from build123d import *

# Parameters (mm, degrees)
BOSS_EXTRUDE1_DEPTH             = 2.54
BOSS_EXTRUDE1_DEPTH_BACK        = 2.54
BOSS_EXTRUDE2_REACH             = 44.034
SKETCH2_R                       = 6.35
BOSS_EXTRUDE2_DIRECTION_2_DEPTH = 1.016
BOSS_EXTRUDE3_DEPTH             = 1.016
BOSS_EXTRUDE3_DEPTH_BACK        = 4.7625
SKETCH3_R                       = 6.35
CUT_EXTRUDE1_DEPTH              = 46.159171383
CUT_EXTRUDE1_DEPTH_BACK         = 46.159171383
BOSS_EXTRUDE4_DEPTH             = 6.35
BOSS_EXTRUDE4_DEPTH_BACK        = 6.35
CUT_EXTRUDE2_DEPTH              = 46.159171383
CUT_EXTRUDE2_DEPTH_BACK         = 46.159171383
SKETCH7_R                       = 0.79375
FILLET1_R                       = 12.7
FILLET2_R                       = 15.875
FILLET3_R                       = 25.4
CUT_EXTRUDE3_DEPTH              = 39.905968649
CUT_EXTRUDE3_DEPTH_BACK         = 39.905968649
SKETCH8_R                       = 2.413


with BuildPart() as part:
    # Sketch1 → Boss-Extrude1 (new, two sides: drawn at the far end of the back side and taken through both)
    with BuildSketch(Plane(origin=(0, 0, 0), x_dir=(1, 0, 0), z_dir=(0, 1, 0)).offset(-BOSS_EXTRUDE1_DEPTH_BACK)):
        with BuildLine():
            Line((-13.716, 6.35), (-8.9535, 6.35))
            Line((-8.9535, 6.35), (-8.9535, -9.525))
            Line((-8.9535, -9.525), (-2.772279089, -20.597609011))
            ThreePointArc((-2.772279089, -20.597609011), (0, -22.225), (2.772279089, -20.597609011))
            Line((2.772279089, -20.597609011), (8.9535, -9.525))
            Line((8.9535, -9.525), (8.9535, 6.35))
            Line((8.9535, 6.35), (13.716, 6.35))
            Line((13.716, 6.35), (13.716, -15.944447946))
            Line((13.716, -15.944447946), (4.32475538, -32.767270057))
            ThreePointArc((4.32475538, -32.767270057), (0, -35.306), (-4.32475538, -32.767270057))
            Line((-4.32475538, -32.767270057), (-13.716, -15.944447946))
            Line((-13.716, -15.944447946), (-13.716, 6.35))
        make_face()
    extrude(amount=BOSS_EXTRUDE1_DEPTH + BOSS_EXTRUDE1_DEPTH_BACK)

    # Boss-Extrude2: up to this face of the body (flat: up to its plane)
    boss_extrude2_end = Plane(part.part.faces().sort_by_distance((-13.716, 0, 4.797223973))[0])
    # Sketch2 → Boss-Extrude2 (add, up to the picked face)
    with BuildSketch(Plane(origin=(-8.9535, 0, 0), x_dir=(0, 0, -1), z_dir=(1, 0, 0)), mode=Mode.PRIVATE) as boss_extrude2_sk1:
        Circle(SKETCH2_R)
    boss_extrude2_tool1 = split(extrude(boss_extrude2_sk1.sketch, amount=-BOSS_EXTRUDE2_REACH, mode=Mode.PRIVATE), bisect_by=boss_extrude2_end, keep=Keep.BOTH, mode=Mode.PRIVATE)
    add(boss_extrude2_tool1.solids().sort_by(Axis((-8.9535, 0, 0), (-1, 0, 0)))[0])

    # Sketch2 → Boss-Extrude2 direction 2 (add)
    with BuildSketch(Plane(origin=(-8.9535, 0, 0), x_dir=(0, 0, -1), z_dir=(1, 0, 0))):
        Circle(SKETCH2_R)
    extrude(amount=BOSS_EXTRUDE2_DIRECTION_2_DEPTH)

    # Sketch3 → Boss-Extrude3 (add, two sides: drawn at the far end of the back side and taken through both)
    with BuildSketch(Plane.ZY.offset(-8.9535).offset(-BOSS_EXTRUDE3_DEPTH_BACK)):
        with Locations(Location((0, 0, 0), (0, 0, 180))):
            Circle(SKETCH3_R)
    extrude(amount=BOSS_EXTRUDE3_DEPTH + BOSS_EXTRUDE3_DEPTH_BACK)

    # Sketch4 → Cut-Extrude1 (cut, two sides: drawn at the far end of the back side and taken through both)
    with BuildSketch(Plane(origin=(13.716, 0, 0), x_dir=(0, 0, -1), z_dir=(1, 0, 0)).offset(-CUT_EXTRUDE1_DEPTH_BACK)):
        with BuildLine():
            Line((3.81, 5.08), (13.97, 5.08))
            Line((13.97, 5.08), (13.97, -5.08))
            Line((13.97, -5.08), (3.81, -5.08))
            ThreePointArc((3.81, -5.08), (6.35, 0), (3.81, 5.08))
        make_face()
    extrude(amount=CUT_EXTRUDE1_DEPTH + CUT_EXTRUDE1_DEPTH_BACK, mode=Mode.SUBTRACT)

    # Sketch6 → Boss-Extrude4 (add, two sides: drawn at the far end of the back side and taken through both)
    with BuildSketch(Plane(origin=(0, 0, 0), x_dir=(1, 0, 0), z_dir=(0, 1, 0)).offset(-BOSS_EXTRUDE4_DEPTH_BACK)):
        with BuildLine():
            Line((-8.9535, -9.525), (-2.772279089, -20.597609011))
            ThreePointArc((-2.772279089, -20.597609011), (0, -22.225), (2.772279089, -20.597609011))
            Line((2.772279089, -20.597609011), (8.9535, -9.525))
            Line((8.9535, -9.525), (8.9535, 0))
            Line((8.9535, 0), (12.1285, 0))
            Line((12.1285, 0), (12.1285, -10.351202795))
            Line((12.1285, -10.351202795), (5.544558179, -22.145218022))
            ThreePointArc((5.544558179, -22.145218022), (0, -25.4), (-5.544558179, -22.145218022))
            Line((-5.544558179, -22.145218022), (-12.1285, -10.351202795))
            Line((-12.1285, -10.351202795), (-12.1285, 0))
            Line((-12.1285, 0), (-8.9535, 0))
            Line((-8.9535, 0), (-8.9535, -9.525))
        make_face()
    extrude(amount=BOSS_EXTRUDE4_DEPTH + BOSS_EXTRUDE4_DEPTH_BACK)

    # Sketch7 → Cut-Extrude2 (cut, two sides: drawn at the far end of the back side and taken through both)
    with BuildSketch(Plane(origin=(13.716, 0, 0), x_dir=(0, 0, -1), z_dir=(1, 0, 0)).offset(-CUT_EXTRUDE2_DEPTH_BACK)):
        Circle(SKETCH7_R)
    extrude(amount=CUT_EXTRUDE2_DEPTH + CUT_EXTRUDE2_DEPTH_BACK, mode=Mode.SUBTRACT)

    # Fillet1
    fillet1_edges = [part.edges().sort_by_distance(p)[0] for p in [
        (-8.9535, 0, 9.525),
        (8.9535, 0, 9.525),
    ]]
    fillet(fillet1_edges, radius=FILLET1_R)

    # Fillet2
    fillet2_edges = [part.edges().sort_by_distance(p)[0] for p in [
        (-12.1285, -4.445, 10.351202795),
        (12.1285, -4.445, 10.351202795),
        (-12.1285, 4.445, 10.351202795),
        (12.1285, 4.445, 10.351202795),
    ]]
    fillet(fillet2_edges, radius=FILLET2_R)

    # Fillet3
    fillet3_edges = [part.edges().sort_by_distance(p)[0] for p in [
        (13.716, 0, 15.944447946),
        (-13.716, 0, 15.944447946),
    ]]
    fillet(fillet3_edges, radius=FILLET3_R)

    # Sketch8 → Cut-Extrude3 (cut, two sides: drawn at the far end of the back side and taken through both)
    with BuildSketch(Plane(origin=(0, 2.54, 0), x_dir=(1, 0, 0), z_dir=(0, 1, 0)).offset(-CUT_EXTRUDE3_DEPTH_BACK)):
        with Locations(Location((0, -30.353, 0), (0, 0, 270))):
            Circle(SKETCH8_R)
    extrude(amount=CUT_EXTRUDE3_DEPTH + CUT_EXTRUDE3_DEPTH_BACK, mode=Mode.SUBTRACT)


solid = part.part
Input: part model. Units: mm. Frame: model coordinates. A direction names the side the tool comes from. Round coordinates to 2 decimals unless told otherwise and drop trailing zeros. Write each loop counter-clockwise with the first axis right and the second up, starting at its lowest first coordinate (ties: lowest second). Pieces come first, ordered by that corner, then holes.
1) Cut plane C-C (x = 6.5). Return the cut outline in (y, z), then the cut area to 3 significant figures.
2) Draft query along Y for faces 1 (the flat face through (-8.954, 5, 5)), 2 (the cylindrical face through (-10.867, -0.775, 0.172)), 3 (the flat face through (0, -2.54, 26)). Return one class per face: pulls with the +Y half, pulls with the -Y half, needs draft (parallel to the pull), parting line crosses it, or undercut.
3) Cut plane B-B (z = 14.5). Return the cut outline in (x, y), then the cut area to 3 significant figures.
4) Reachability of faces 4 (the cylindrical face through (-11.63, -4.42, 10.16)), 5 (the flat face through (-5.09, -0.089, 16.445)), 6 (the flat face through (-8.954, -5, 5)), 7 (the flat face through (8.954, 5, 5)) from +Z, -Z, +X, -X, +Y, -Y: full face, straight path, thin tool, end or side. Return the list, or none.
5) Contact query for a flat-ended pin moving along its axis: P1, Ø2, axis at x = 6, z = 24.5, coming from the -Y side. Output: stop coordinate, or through.
6) Cut plane A-A (x = 0). Return the cut outline in (y, z) (3 decimals), then the cut area to 3 significant figures.
7) Ray query, L1, parallel to Z at x = 10.25, y = 0; L2, parallel to X at y = -1.75, z = 4; L3, parallel to Z at x = 0, y = 1.15 (3 decimals). Return the intervals inside material, ascending.
Geometry says:
1. outline: (-6.35, 13.92) - (6.35, 13.92) - (6.35, 20.43) - (2.54, 20.43) - (2.54, 28.87) - (-2.54, 28.87) - (-2.54, 20.43) - (-6.35, 20.43) - close
1. area: 126 mm2
2. face 1: needs draft
2. face 2: undercut
2. face 3: pulls with the -Y half
3. outline: (-13.19, -2.54) - (-9.81, -2.54) - (-9.81, -6.35) - (-6.18, -6.35) - (-6.18, 6.35) - (-9.81, 6.35) - (-9.81, 2.54) - (-13.19, 2.54) - close; (6.18, -6.35) - (9.81, -6.35) - (9.81, -2.54) - (13.19, -2.54) - (13.19, 2.54) - (9.81, 2.54) - (9.81, 6.35) - (6.18, 6.35) - close
3. area: 127 mm2
4. face 4: +Z, -X, -Y
4. face 5: -Z, +Y, -Y
4. face 6: -Y
4. face 7: +Y
5. P1: stops at y = -2.54
6. outline: (-6.35, 22.225) - (6.35, 22.225) - (6.35, 25.4) - (2.54, 25.4) - (2.54, 27.94) - (-2.54, 27.94) - (-2.54, 25.4) - (-6.35, 25.4) - close; (-2.54, 32.766) - (2.54, 32.766) - (2.54, 35.306) - (-2.54, 35.306) - close
6. area: 66.1 mm2
7. L1: z = -6.35 to -0.79, 0.79 to 22.15
7. L2: x = -13.72 to -7.94, 7.94 to 13.72
7. L3: z = 22.225 to 27.94, 32.766 to 35.306
